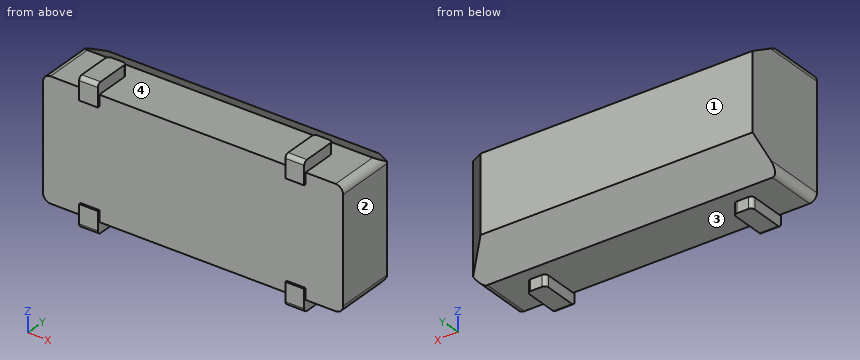
from build123d import *

# Parameters (mm, degrees)
SKETCH_1_W             = 8
SKETCH_1_H             = 3.2
EXTRUDE_1_DEPTH        = 2.35
SKETCH_2_W             = 0.5
SKETCH_2_H             = 0.6
EXTRUDE_2_DEPTH        = 0.05
EXTRUDE_2_DEPTH_BACK   = 1
FILLET_1_R             = 0.1
CHAMFER_1_SIZE         = 1
CHAMFER_1_SIZE2        = 0.577350269
CHAMFER_1_PART_2_SIZE  = 1
CHAMFER_1_PART_2_SIZE2 = 0.577350269
CHAMFER_2_SIZE         = 0.75
FILLET_2_R             = 0.2


with BuildPart() as part:
    # Эскиз1 → Бобышка-Вытянуть1 (new body)
    with BuildSketch(Plane(origin=(0, 0, 0), x_dir=(1, 0, 0), z_dir=(0, 1, 0))):
        Rectangle(SKETCH_1_W, SKETCH_1_H)
    extrude(amount=EXTRUDE_1_DEPTH)

    # Эскиз2 → Бобышка-Вытянуть2 (add, two sides)
    with BuildSketch(Plane.XZ) as extrude_2_sk:
        with Locations((-2.75, 1.6)):
            Rectangle(SKETCH_2_W, SKETCH_2_H)
        with Locations((2.75, 1.6)):
            Rectangle(SKETCH_2_W, SKETCH_2_H)
        with Locations((2.75, -1.6)):
            Rectangle(SKETCH_2_W, SKETCH_2_H)
        with Locations((-2.75, -1.6)):
            Rectangle(SKETCH_2_W, SKETCH_2_H)
    extrude(amount=EXTRUDE_2_DEPTH)
    extrude(extrude_2_sk.sketch, amount=-EXTRUDE_2_DEPTH_BACK)

    # Скругление1
    fillet_1_edges = [part.edges().sort_by_distance(p)[0] for p in [
        (-2.5, 1, 1.75),
        (-3, 1, 1.75),
        (-2.75, -0.05, 1.9),
        (3, 1, 1.75),
        (2.5, 1, 1.75),
        (2.75, -0.05, 1.9),
        (3, 1, -1.75),
        (2.5, 1, -1.75),
        (2.75, -0.05, -1.9),
        (-3, 1, -1.75),
        (-2.5, 1, -1.75),
        (-2.75, -0.05, -1.9),
    ]]
    fillet(fillet_1_edges, radius=FILLET_1_R)

    # Фаска1
    chamfer_1_edges = [part.edges().sort_by_distance(p)[0] for p in [
        (0, 2.35, 1.6),
    ]]
    chamfer_1_side = [part.faces().sort_by_distance(p)[0] for p in [
        (0, 1.212807949, 1.6),
    ]]
    chamfer(chamfer_1_edges, length=CHAMFER_1_SIZE, length2=CHAMFER_1_SIZE2, reference=chamfer_1_side[0])

    # Фаска1 part 2
    chamfer_1_part_2_edges = [part.edges().sort_by_distance(p)[0] for p in [
        (0, 2.35, -1.6),
    ]]
    chamfer_1_part_2_side = [part.faces().sort_by_distance(p)[0] for p in [
        (0, 1.212807949, -1.6),
    ]]
    chamfer(chamfer_1_part_2_edges, length=CHAMFER_1_PART_2_SIZE, length2=CHAMFER_1_PART_2_SIZE2, reference=chamfer_1_part_2_side[0])

    # Фаска2
    chamfer_2_edges = [part.edges().sort_by_distance(p)[0] for p in [
        (4, 2.35, 0),
    ]]
    chamfer(chamfer_2_edges, length=CHAMFER_2_SIZE)

    # Скругление2
    fillet_2_edges = [part.edges().sort_by_distance(p)[0] for p in [
        (-4, 0.675, 1.6),
        (-4, 0.675, -1.6),
        (4, 0.675, 1.6),
        (4, 0.675, -1.6),
    ]]
    fillet(fillet_2_edges, radius=FILLET_2_R)


solid = part.part
Check sheet for the modelled part. Datum: model origin and axes. Units: mm. Face numbers are marked on the shaded views. Give positions to 0.01 mm unless a question says otherwise; leave off trailing zeros. Order: outer loops, then holes, each group sorted by start corner. A loop starts at its lowest first (then second) coordinate and runs counter-clockwise, first axis right, second up. Notation, with made-up numbers: (-1, 89.5) - (26, 89.5) arc R20 cw to (26, 111.5) - close; hole circle Ø6 at (-29.5, 79.5). An arc over 180 degrees is marked (long way). Answer as CSV lines item,"result".
1. Section check A-A (x = -0.25). Record the boundary of the cut face in (y, z), then the cut area to 3 significant figures.
Result sheet:
outline,"(0, -1.6) - (1.35, -1.6) - (2.35, -1.02) - (2.35, 1.02) - (1.35, 1.6) - (0, 1.6) - close"
area,"6.94 mm²"
2. Scan lines: probe 1 along Z at (x, y) = (3.5, 1); probe 2 along Y at (x, z) = (-2.75, 0.25); probe 3 along X at (y, z) = (1.8, -0.65). Record each from-to range of solid material in increasing order. Write a range as from..to.
Result sheet:
probe 1,"-1.6..1.6"
probe 2,"0..2.35"
probe 3,"-4..3.8"
3. Go/stop test with flat-tipped pins: P1, Ø0.7, axis at y = 0.5, z = 1.5, coming from the +X side; P2, Ø1, axis at x = 1.5, y = 1.5, coming from the -Z side; P3, Ø1.5, axis at x = 0, z = 1, coming from the -Y side. Record where each tip stops, or that it passes through.
Result sheet:
P1,"x = 4"
P2,"z = -1.6"
P3,"y = 0"
4. Section check D-D (z = 1.2). Record the boundary of the cut face in (x, y), then the cut area to 3 significant figures.
Result sheet:
outline,"(-4, 0) - (4, 0) - (4, 1.6) - (3.56, 2.04) - (-4, 2.04) - close"
area,"16.2 mm²"
5. Section check B-B (z = 0.3). Record the boundary of the cut face in (x, y).
Result sheet:
outline,"(-4, 0) - (4, 0) - (4, 1.6) - (3.25, 2.35) - (-4, 2.35) - close"
6. Mould release check, pull along X, two halves, no side actions. Record for the marked faces 1, 2, 3 and 4: released by +X, released by -X, zero draft, split by the parting line, or undercut.
Result sheet:
face 1,"zero draft"
face 2,"released by +X"
face 3,"undercut"
face 4,"undercut"
7. Section check C-C (y = 1.8). Record the boundary of the cut face in (x, z).
Result sheet:
outline,"(-4, -1.34) - (3.8, -1.34) - (3.8, 1.34) - (-4, 1.34) - close"
